Here's how the part is built. I have some questions about the finished solid (model axes, mm). A direction names the side the tool comes from. Give positions to 0.01 mm unless a question says otherwise; leave off trailing zeros. Loops run counter-clockwise (first coordinate to the right, second up) from the corner with the lowest first, then second, coordinate; pieces in that order, holes last. Notation, with made-up numbers: (43, 38.5) -> (93, 38.5) arc R22 ccw to (93, 75.5) -> close; hole circle Ø9 at (45.5, 47.5). An arc over 180 degrees is marked (long way). Answer in a Markdown table with one row per item. Add a question column.
Item 1: If we section it at B-B (z = -17.5): Write out the boundary of the cut face in (x, y).
Item 2: If we section it at C-C (y = 18.5): Write out the boundary of the cut face in (x, z).
Item 3: If we section it at D-D (x = 1): Write out the boundary of the cut face in (y, z).
Item 4: If I drill on line 1 (Y direction, x = 4, z = 17); line 2 (Z direction, x = 4, y = 7); line 3 (Z direction, x = 4, y = 5.75), over which ranges is the centre line in solid material (lowest first)?
Item 5: We'd pull the mould along X, two halves only. Please class faces 1 (the face through (4.06, 5.04, 20.25)), 2 (the face through (4.009, 20.61, -22.787)), 3 (the face through (8, 34, 0)), 4 (the face through (4.471, 10.14, -24.136)): released by +X, released by -X, zero draft, split by the parting line, or undercut.
Item 6: For P1, Ø2, axis at x = 6, z = 15, coming from the -Y side; P2, Ø2, axis at x = 4, z = 22, coming from the -Y side, each with a flat end and sliding along its axis, tell me the tip position at first contact or that it passes through.
Item 7: If we section it at A-A (y = 5): Write out the boundary of the cut face in (x, z), then the cut area to 3 significant figures.
Item 8: Which directions (+Z, -Z, +X, -X, +Y, -Y) give clear straight access to the entire face, cutting with the end or side of a thin tool? Please do faces 5 (the face through (4, 39, 25)), 6 (the face through (4.471, 10.14, 20.864)), 7 (the face through (4, 34.25, -16)).
Autodesk Inventor part; units mm, degrees
ref_plane "YZ Plane" through (0, 0, 0) normal (1, 0, 0) x (0, 1, 0)
ref_plane "XZ Plane" through (0, 0, 0) normal (0, 1, 0) x (-1, 0, 0)
ref_plane "XY Plane" through (0, 0, 0) normal (0, 0, 1) x (1, 0, 0)
sketch "Sketch1" plane through (0, 0, 0) normal (0, 1, 0) x (-1, 0, 0)
  line L0 (0, 0) -> (-8, 0)
  line L1 (-8, 0) -> (-8, -27)
  line L2 (-8, -27) -> (0, -27)
  line L3 (0, -27) -> (0, 0)
  line L4 (0, 0) -> (-8, 0)
  line L5 (-8, 0) -> (-8, 26)
  line L6 (-8, 26) -> (0, 26)
  line L7 (0, 26) -> (0, 0)
  dimension "d0" = 8
  dimension "d3" = 27
  dimension "d4" = 26
extrude "Extrusion1" add sketch "Sketch1" along normal blind 41
sketch "Sketch2" plane through (8, 0, 26) normal (1, 0, 0) x (0, 0, -1)
  circle A0 centre (26.5, 20.5) radius 7.5
  circle A1 centre (11, 36) radius 1.5
  circle A2 centre (11, 5) radius 1.5
  circle A3 centre (42, 36) radius 1.5
  circle A4 centre (42, 5) radius 1.5
  arc A5 (14.5, 34.25) -> (14.5, 37.75) centre (14.5, 36) ccw
  arc A6 (7.5, 37.75) -> (7.5, 34.25) centre (7.5, 36) ccw
  line L0 (2.4202, 36) -> (21.3421, 36) construction
  arc A7 (23.5, 32.5) -> (23.5, 8.5) centre (23.5, 20.5) ccw
  arc A8 (29.5, 8.5) -> (29.5, 32.5) centre (29.5, 20.5) ccw
  line L1 (12.5, 20.5) -> (42, 20.5) construction
  line L2 (26.5, 35.5013) -> (26.5, 5.593) construction
  circle A9 centre (42, 36) radius 1.5
  arc A10 (38.5, 37.75) -> (38.5, 34.25) centre (38.5, 36) ccw
  arc A11 (45.5, 34.25) -> (45.5, 37.75) centre (45.5, 36) ccw
  line L3 (45.5, 37.75) -> (38.5, 37.75)
  line L4 (38.5, 34.25) -> (45.5, 34.25)
  circle A12 centre (11, 5) radius 1.5
  circle A13 centre (42, 5) radius 1.5
  arc A14 (14.5, 3.25) -> (14.5, 6.75) centre (14.5, 5) ccw
  arc A15 (7.5, 6.75) -> (7.5, 3.25) centre (7.5, 5) ccw
  line L5 (7.5, 3.25) -> (14.5, 3.25)
  line L6 (14.5, 6.75) -> (7.5, 6.75)
  line L7 (2.4202, 5) -> (21.3421, 5) construction
  circle A16 centre (42, 5) radius 1.5
  arc A17 (38.5, 6.75) -> (38.5, 3.25) centre (38.5, 5) ccw
  line L8 (38.5, 6.75) -> (45.5, 6.75)
  line L9 (45.5, 3.25) -> (38.5, 3.25)
  arc A18 (45.5, 3.25) -> (45.5, 6.75) centre (45.5, 5) ccw
  line L10 (23.5, 32.5) -> (29.5, 32.5)
  line L11 (23.5, 8.5) -> (29.5, 8.5)
  line L12 (7.5, 37.75) -> (14.5, 37.75)
  line L13 (14.5, 34.25) -> (7.5, 34.25)
  point P0 (26, 0)
  point P1 (50.5798, 36)
  point P2 (26.5, 5.4987)
  point P3 (50.5798, 5)
  point P4 (11, 3.5)
  point P5 (11, 6.5)
  point P6 (42, 6.5)
  point P7 (42, 3.5)
  point P8 (42, 37.5)
  point P9 (42, 34.5)
  dimension "d8" = 3.5
  dimension "d9" = 3.5
  dimension "d10" = 3.5
  dimension "d11" = 3.5
  dimension "d14" = 3
  dimension "d15" = 3
  dimension "d16" = 12
  dimension "d17" = 12
  dimension "d33" = 3.5
extrude "Extrusion2" cut sketch "Sketch2" against normal blind 10 contours A0 | A1 | A2 | A3 | A4 | L13 A6 L12 A5 | L10 A8 L11 A7 | L3 A11 L4 A10 | L5 A15 L6 A14 | L8 A18 L9 A17
fillet "Fillet1" radius 5 2 edges at (4, 41, 26) (4, 41, -27)
sketch "Sketch3" plane through (0, 0, 0) normal (0, -1, 0) x (1, 0, 0)
  line L0 (4, 28.9228) -> (4, -37.7056) construction
  circle A0 centre (4, 22) radius 1.5
  circle A1 centre (4, -23) radius 1.5
  circle A2 centre (4, 0) radius 1.5
  line L1 (8, 26) -> (8, -27)
  line L2 (0, 26) -> (8, 26)
  line L3 (8, -27) -> (0, -27)
  point P0 (0, 0)
  dimension "d20" = 3
  dimension "d21" = 3
  dimension "d22" = 3
  dimension "d23" = 4
  dimension "d24" = 4
  dimension "d25" = 4
hole "Hole2" at (4, 0, 22) at (4, 0, 0) at (4, 0, -23) direction (0, 1, 0) diameter 2.459 depth 20 tip angle 118
properties part number "Z_Motorhalter_oben"
Recorded:
| question | item | result |
|---|---|---|
| 1 | outline | (0, 0) -> (8, 0) -> (8, 3.25) -> (0, 3.25) -> close; (0, 6.75) -> (8, 6.75) -> (8, 34.25) -> (0, 34.25) -> close; (0, 37.75) -> (8, 37.75) -> (8, 41) -> (0, 41) -> close |
| 2 | outline | (0, -27) -> (8, -27) -> (8, -15.33) -> (0, -15.33) -> close; (0, 14.33) -> (8, 14.33) -> (8, 26) -> (0, 26) -> close; hole circle Ø2.46 at (4, -23); hole circle Ø2.46 at (4, 22) |
| 3 | outline | (0, -27) -> (36, -27) arc R5 ccw to (41, -22) -> (41, 21) arc R5 ccw to (36, 26) -> (0, 26) -> close; hole (3.25, -19.5) arc R1.75 ccw to (6.75, -19.5) -> (6.75, -12.5) arc R1.75 ccw to (3.25, -12.5) -> close; hole (3.25, 11.5) arc R1.75 ccw to (6.75, 11.5) -> (6.75, 18.5) arc R1.75 ccw to (3.25, 18.5) -> close; hole (8.5, -3.5) arc R12 ccw to (32.5, -3.5) -> (32.5, 2.5) arc R12 ccw to (8.5, 2.5) -> close; hole (34.25, -19.5) arc R1.75 ccw to (37.75, -19.5) -> (37.75, -12.5) arc R1.75 ccw to (34.25, -12.5) -> close; hole (34.25, 11.5) arc R1.75 ccw to (37.75, 11.5) -> (37.75, 18.5) arc R1.75 ccw to (34.25, 18.5) -> close |
| 4 | line 1 | y = 0 to 3.25, 6.75 to 34.25, 37.75 to 41 |
| 4 | line 2 | z = -27 to -24.23, -21.77 to -1.23, 1.23 to 20.77, 23.23 to 26 |
| 4 | line 3 | z = -27 to -24.23, -21.77 to -21.08, -10.92 to -1.23, 1.23 to 9.92, 20.08 to 20.77, 23.23 to 26 |
| 5 | face 1 | zero draft |
| 5 | face 2 | undercut |
| 5 | face 3 | released by +X |
| 5 | face 4 | undercut |
| 6 | P1 | stops at y = 0 |
| 6 | P2 | stops at y = 20.14 |
| 7 | outline | (0, -27) -> (8, -27) -> (8, -21.25) -> (0, -21.25) -> close; (0, -10.75) -> (8, -10.75) -> (8, 9.75) -> (0, 9.75) -> close; (0, 20.25) -> (8, 20.25) -> (8, 26) -> (0, 26) -> close; hole circle Ø2.46 at (4, -23); hole circle Ø2.46 at (4, 0); hole circle Ø2.46 at (4, 22) |
| 7 | area | 242 mm^2 |
| 8 | face 5 | +Z, +X, -X, +Y |
| 8 | face 6 | -Y |
| 8 | face 7 | +X, -X |
